Input: part model. Units: mm. Frame: model coordinates. Round coordinates to 2 decimals unless told otherwise and drop trailing zeros. Write each loop counter-clockwise with the first axis right and the second up, starting at its lowest first coordinate (ties: lowest second). Pieces come first, ordered by that corner, then holes. Notation, with made-up numbers: M 77.25,11 L 103.25,11 A20 cw 103.25,43 Z; hole C 43,-5.5 d7. An arc over 180 degrees is marked long. Write each question's results on one line, items separated by ' | '. Start each with the question number.
Autodesk Inventor part; units mm, degrees
ref_plane "MountPlane" through (0, -10, 0) normal (0, -1, 0) x (1, 0, 0)
ref_plane "YZ Plane" through (0, 0, 0) normal (1, 0, 0) x (0, 1, 0)
ref_plane "XY Plane" through (0, 0, 0) normal (0, 0, 1) x (1, 0, 0)
sketch "Base" plane through (0, 0, 0) normal (0, 0, 1) x (1, 0, 0)
  circle A0 centre (0, 0) radius 9.525
  dimension "d0" = 19.05
extrude "BaseFeature" add sketch "Base" along normal blind 117.475
chamfer "BaseChamferFeature" distance 0.508 angle 45 1 edges at (-9.525, 0, 117.475)
sketch "MountHole" plane through (0, 0, 0) normal (0, 1, 0) x (-1, 0, 0)
  line L0 (-9.017, 117.475) -> (9.017, 117.475) construction
  line L1 (0, 117.475) -> (0, 111.633) construction
  line L2 (0, 111.633) -> (0, 107.95) construction
  circle A0 centre (0, 107.95) radius 3.683
  point P0 (0, 0)
  dimension "d6" = 5.842
  dimension "d7" = 3.683
extrude "MountHoleFeature" cut sketch "MountHole" along normal through all both and the other way through all
chamfer "MountHoleChamferFeature" distance 0.507 angle 45 2 edges at (3.683, -8.7841, 107.9534) (3.683, 8.7841, 107.9534)
ref_plane "MountPlane" through (0, -10, 0) normal (0, -1, 0) x (1, 0, 0)
properties part number "FA-RMS-15-12-4-Piston"
1. Draft query along X for faces 1 (the face through (9.085, -2.861, 57.665)), 2 (the face through (0, 0, 0)), 3 (the face through (2.715, -0.126, 105.461)). Return one class per face: +X half, -X half, draft (parallel to the pull), parting line (faces both ways), or undercut.
2. Line query: L1, parallel to X at y = -0.25, z = 107.95; L2, parallel to Z at x = 0, y = 4 (3 decimals); L3, parallel to X at y = 4.25, z = 107.95. Output: solid intervals per line, ascending. Write a range as from..to.
3. Contact query for flat-ended pins moving along their axis: P1, Ø2, axis at x = -7.5, z = 77, coming from the +Y side; P2, Ø5, axis at y = 6.5, z = 93, coming from the +X side; P3, Ø5, axis at x = -6.5, z = 65, coming from the -Y side; P4, Ø4.5, axis at x = 0, z = 107.95, coming from the -Y side. Output: stop coordinate, or through.
4. Cut plane B-B on z = 78. Output: boundary loops of the cut face in (x, y) (3 decimals), and give its area (3 significant figures).
5. Cut plane A-A on y = 0. Output: boundary loops of the cut face in (x, z) (3 decimals), and give its area (3 significant figures).
Answers follow:
1) face 1: parting line | face 2: draft | face 3: undercut
2) L1: x = -9.52..-3.68, 3.68..9.52 | L2: z = 0..104.267, 111.633..117.475 | L3: x = -8.52..-3.68, 3.68..8.52
3) P1: stops at y = 6.96 | P2: stops at x = 8.64 | P3: stops at y = -8.64 | P4: passes through
4) outline: C 0,0 d19.05 | area: 285 mm2
5) outline: M -9.525,0 L 9.525,0 L 9.525,116.967 L 9.017,117.475 L -9.017,117.475 L -9.525,116.967 Z; hole C 0,107.95 d7.366 | area: 2,200 mm2
